Geometry check sheet. Reference: the model listing, model coordinates, mm. Round coordinates to 2 decimals unless told otherwise and drop trailing zeros. Loops run counter-clockwise (first coordinate to the right, second up) from the corner with the lowest first, then second, coordinate; pieces in that order, holes last. Notation, with made-up numbers: (87, 38) - (102, 38) arc R19 cw to (102, 52) - close; hole circle Ø3 at (-14.75, 24). An arc over 180 degrees is marked (long way). Answer in a Markdown table with one row per item. Add a question column.
Autodesk Inventor part; units mm, degrees
ref_plane "YZ Plane" through (0, 0, 0) normal (1, 0, 0) x (0, 1, 0)
ref_plane "XZ Plane" through (0, 0, 0) normal (0, 1, 0) x (-1, 0, 0)
ref_plane "XY Plane" through (0, 0, 0) normal (0, 0, 1) x (1, 0, 0)
sketch "Sketch1" plane through (0, 0, 0) normal (0, 0, 1) x (1, 0, 0)
  line L0 (66.7253, 90.1264) -> (-18.9997, 90.1264)
  line L1 (-18.9997, 90.1264) -> (-18.9997, 52.0264)
  line L2 (-18.9997, 52.0264) -> (66.7253, 52.0264)
  line L3 (66.7253, 52.0264) -> (66.7253, 90.1264)
  line L4 (66.7253, 78.1884) -> (-18.9997, 78.1884)
  line L5 (-18.9997, 78.1884) -> (-18.9997, 76.5584)
  line L6 (-18.9997, 76.5584) -> (66.7253, 76.5584)
  line L7 (66.7253, 76.5584) -> (66.7253, 78.1884)
  line L8 (55.9303, 78.1884) -> (55.9303, 76.5584)
  line L9 (-11.3797, 76.5584) -> (-11.3797, 78.1884)
  point P0 (0, 0)
  dimension "d0" = 38.1
  dimension "d1" = 85.725
  dimension "d2" = 1.63
  dimension "d3" = 11.938
  dimension "d6" = 67.31
  dimension "d7" = 7.62
extrude "Extrusion1" add sketch "Sketch1" along normal blind 3.175 contours L3 L4 L1 L0 | L3 L6 L8 L4 | L4 L9 L6 L1 | L3 L2 L1 L6
sketch "Sketch2" plane through (0, 0, 0) normal (0, 0, -1) x (-1, 0, 0)
  line L0 (-55.9303, 78.1884) -> (11.3797, 78.1884)
  line L1 (-6.3913, 84.1043) -> (3.1337, 84.1043)
  line L2 (3.1337, 84.1043) -> (3.1337, 74.5793)
  line L3 (3.1337, 74.5793) -> (-6.3913, 74.5793)
  line L4 (-6.3913, 74.5793) -> (-6.3913, 84.1043)
  line L5 (-39.708, 84.1761) -> (-30.183, 84.1761)
  line L6 (-30.183, 84.1761) -> (-30.183, 74.6584)
  line L7 (-30.183, 74.6584) -> (-39.708, 74.6584)
  line L8 (-39.708, 74.6584) -> (-39.708, 84.1761)
  line L9 (18.9997, 52.0264) -> (-66.7253, 52.0264)
  line L10 (-50.8503, 52.0264) -> (-12.7503, 52.0264)
  line L11 (-66.7253, 90.1264) -> (18.9997, 90.1264)
  line L12 (-28.6253, 90.1264) -> (-15.9253, 90.1264)
  point P0 (0, 0)
  dimension "d8" = 9.525
  dimension "d9" = 9.5177
  dimension "d10" = 9.525
  dimension "d11" = 9.525
  dimension "d13" = 5.9159
extrude "Extrusion2" cut sketch "Sketch2" against normal blind 3.175
properties part number "FrontBulkhead"
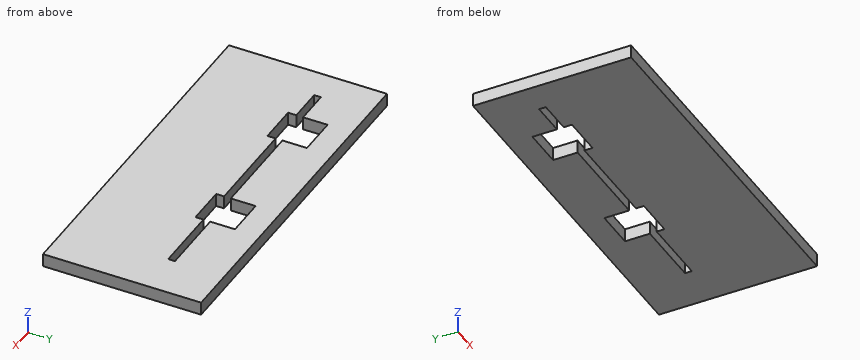
Q1. Cross-section at B-B, the plane x = 40.5. Enter the section's corners in (y, z) (3 decimals).
Q2. Depth check by flat-ended pin: P1, Ø8, axis at x = 26.5, y = 81.5, coming from the -Z side. Enter the tip coordinate at first touch or a pass-through.
Q3. Scan lines: line 1 (X direction, y = 82, z = 1.95); line 2 (Y direction, x = 28.5, z = 0.95); line 3 (Y direction, x = 34, z = 3.05). Record each from-to range of solid material in increasing order. Write a range as from..to.
Q4. Cross-section at A-A, the plane z = 1.6. Enter the section's corners in (x, y).
Check sheet entries:
| question | item | result |
|---|---|---|
| 1 | outline | (52.026, 0) - (76.558, 0) - (76.558, 3.175) - (52.026, 3.175) - close; (78.188, 0) - (90.126, 0) - (90.126, 3.175) - (78.188, 3.175) - close |
| 2 | P1 | z = 0 |
| 3 | line 1 | -19..-3.13, 6.39..30.18, 39.71..66.73 |
| 3 | line 2 | 52.03..76.56, 78.19..90.13 |
| 3 | line 3 | 52.03..74.66, 84.18..90.13 |
| 4 | outline | (-19, 52.03) - (66.73, 52.03) - (66.73, 90.13) - (-19, 90.13) - close; hole (-11.38, 76.56) - (-3.13, 76.56) - (-3.13, 74.58) - (6.39, 74.58) - (6.39, 76.56) - (30.18, 76.56) - (30.18, 74.66) - (39.71, 74.66) - (39.71, 76.56) - (55.93, 76.56) - (55.93, 78.19) - (39.71, 78.19) - (39.71, 84.18) - (30.18, 84.18) - (30.18, 78.19) - (6.39, 78.19) - (6.39, 84.1) - (-3.13, 84.1) - (-3.13, 78.19) - (-11.38, 78.19) - close |
